Geometry: final body of the model. Coordinates: model frame, mm. Face numbers are marked on the shaded views. A direction names the side the tool comes from. Give positions to 0.01 mm unless a question says otherwise; leave off trailing zeros. Write each loop counter-clockwise with the first axis right and the second up, starting at its lowest first coordinate (ties: lowest second). Pieces come first, ordered by that corner, then holes. Notation, with made-up numbers: M 18,28.5 L 46,28.5 A25 cw 46,40.5 Z; hole C 34,89.5 d2. An arc over 180 degrees is marked long. Use a Markdown table: item, result. Add a question column.
(1) Cut plane C-C (z = 2). Output: boundary loops of the cut face in (x, y).
(2) Pin query (flat end, axial travel): pin 1 Ø8 at (x, z) = (24.5, 19.5) entering from -Y; pin 2 Ø6 at (x, y) = (-22.5, 1.5) entering from -Z; pin 3 Ø23 at (x, y) = (12.6, 12.6) entering from -Z; pin 4 Ø10 at (x, y) = (29.5, 5.5) entering from +Z. Return the tip coordinate at first contact, or that it passes through.
(3) Cut plane B-B (x = -23.5). Output: boundary loops of the cut face in (y, z), plus the area to 3 significant figures.
(4) Cut plane D-D (x = 26). Output: boundary loops of the cut face in (y, z).
(5) Material intervals for L1, parallel to Z at x = 11.5, y = -16.5; L2, parallel to Y at x = 14, z = 11.25, sorted ascending.
(6) Reachability of the marked faces 1 and 2 from +Z, -Z, +X, -X, +Y, -Y: full face, straight path, thin tool, end or side. Return the list, or none.
(7) Cut plane A-A (y = 25.5). Output: boundary loops of the cut face in (x, z), plus the area to 3 significant figures.
```python
from build123d import *

# Parameters (mm, degrees)
F1_DEPTH = 3.81
F3_DEPTH = 20.32
F4_R     = 19.05
F5_DEPTH = 39.624


with BuildPart() as f1:
    # F0 (on Top) → F1 (new body)
    with BuildSketch(Plane.XY):
        Polygon((24.13, -44.45), (44.45, -44.45), (44.45, 44.45), (-44.45, 44.45), (-44.45, 24.13), align=None)
    extrude(amount=F1_DEPTH)

    # F2 (on face) → F3 (join)
    with BuildSketch(Plane.XY.offset(3.81)):
        Polygon((40.64, 44.45), (-44.45, 44.45), (-44.45, 40.64), (40.64, 40.64), (40.64, -44.45), (44.45, -44.45), (44.45, 40.64), (44.45, 44.45), align=None)
    extrude(amount=F3_DEPTH)

    # F4 (on face) → F5 (cut)
    with BuildSketch(Plane.XY.offset(3.81)):
        with Locations((12.604465, 12.604465)):
            Circle(F4_R)
    extrude(amount=-F5_DEPTH, mode=Mode.SUBTRACT)


solid = f1.part
```
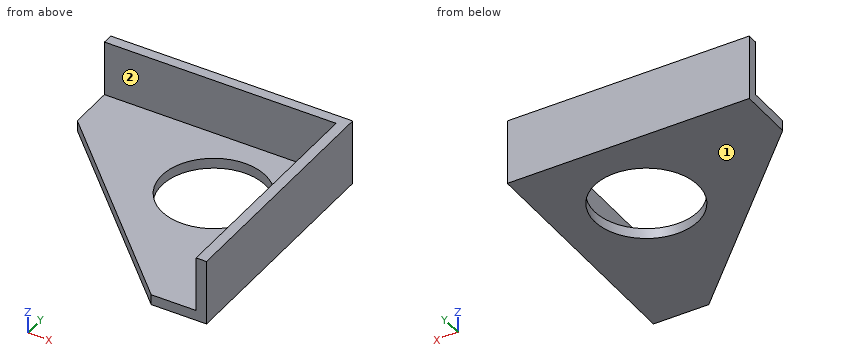
Answer list:
| question | item | result |
|---|---|---|
| 1 | outline | M -44.45,24.13 L 24.13,-44.45 L 44.45,-44.45 L 44.45,44.45 L -44.45,44.45 Z; hole C 12.6,12.6 d38.1 |
| 2 | pin 1 | y = 40.64 |
| 2 | pin 2 | z = 0 |
| 2 | pin 3 | through |
| 2 | pin 4 | z = 3.81 |
| 3 | outline | M 3.18,0 L 44.45,0 L 44.45,24.13 L 40.64,24.13 L 40.64,3.81 L 3.18,3.81 Z |
| 3 | area | 235 mm² |
| 4 | outline | M -44.45,0 L -0.94,0 L -0.94,3.81 L -44.45,3.81 Z; M 26.15,0 L 44.45,0 L 44.45,24.13 L 40.64,24.13 L 40.64,3.81 L 26.15,3.81 Z |
| 5 | L1 | 0 to 3.81 |
| 5 | L2 | 40.64 to 44.45 |
| 6 | face 1 | -Z, +X, -X, +Y, -Y |
| 6 | face 2 | +Z, -X, -Y |
| 7 | outline | M -44.45,0 L -1.42,0 L -1.42,3.81 L -44.45,3.81 Z; M 26.63,0 L 44.45,0 L 44.45,24.13 L 40.64,24.13 L 40.64,3.81 L 26.63,3.81 Z |
| 7 | area | 309 mm² |
